Autodesk Inventor part; units mm, degrees
ref_plane "Płaszczyzna konstrukcyjna1" through (0, 15, 0) normal (0, 1, 0) x (-1, 0, 0)
ref_plane "YZ Plane" through (0, 0, 0) normal (1, 0, 0) x (0, 1, 0)
ref_plane "XY Plane" through (0, 0, 0) normal (0, 0, 1) x (1, 0, 0)
sketch "Szkic1" plane through (0, 0, 0) normal (0, 1, 0) x (-1, 0, 0)
  line L0 (15, 0) -> (-15, 0)
  line L1 (-15, 0) -> (-15, -600)
  line L2 (-15, -600) -> (15, -600)
  line L3 (15, -600) -> (15, 0)
  point P0 (0, 0)
  point P1 (0, 0)
  dimension "d0" = 30
  dimension "d1" = 600
extrude "Wyciągnięcie proste1" add sketch "Szkic1" along normal blind 30
sketch "Szkic2" plane through (-15, 0, 0) normal (0, 0, 1) x (1, 0, 0)
  line L0 (0, 0) -> (0, 30)
  line L1 (0, 0) -> (30, 0)
  line L2 (30, 0) -> (30, 30)
  line L3 (0, 30) -> (30, 30)
  line L4 (0, 0) -> (0, 30)
  line L5 (0, -15) -> (30, -15)
  line L6 (30, -15) -> (30, 45)
  line L7 (30, 45) -> (0, 45)
  line L8 (0, 45) -> (0, -15)
  point P0 (15, 0)
  point P1 (0, 15)
  point P2 (0, 15)
  dimension "d4" = 60
  dimension "d5" = 30
extrude "Wyciągnięcie proste2" add sketch "Szkic2" along normal blind 10
sketch "Szkic3" plane through (-15, 0, 10) normal (0, 0, 1) x (1, 0, 0)
  line L0 (0, -15) -> (30, -15)
  line L1 (30, -15) -> (30, 45)
  line L2 (0, -15) -> (30, -15)
  line L3 (30, -15) -> (30, 0)
  line L4 (30, 0) -> (0, 0)
  line L5 (0, 0) -> (0, -15)
  point P0 (15, 0)
extrude "Wyciągnięcie proste3" add sketch "Szkic3" along normal blind 60
ref_plane "Płaszczyzna konstrukcyjna1" through (0, 15, 0) normal (0, 1, 0) x (-1, 0, 0)
mirror "Odbicie lustrzane1" about plane through (0, 15, 0) normal (0, 1, 0) of "Wyciągnięcie proste3"
sketch "Szkic4" plane through (0, 15, 0) normal (0, 1, 0) x (-1, 0, 0)
  point P0 (0, 0)
sketch "Szkic5" plane through (-15, 45, 0) normal (0, 1, 0) x (1, 0, 0)
  line L0 (0, -70) -> (30, -70)
  line L1 (30, 0) -> (30, -70)
  circle A0 centre (15, -50) radius 7.5
  point P0 (15, 0)
  dimension "d11" = 15
  dimension "d12" = 20
  dimension "d13" = 15
extrude "Wyciągnięcie proste4" cut sketch "Szkic5" against normal through all
fillet "Zaokrąglenie1" radius 4 12 edges at (0, 45, 0) (0, 45, 70) (0, 0, 70) (-15, 0, -300) (-15, 30, -300) (-15, 15, -600) (0, 0, -600) (0, 30, -600) (15, 15, -600) (15, 0, -300) (15, 30, -300) (0, -15, 0)
sketch "Szkic6" plane through (0, 0, 0) normal (0, -1, 0) x (1, 0, 0)
  circle A0 centre (0, -580) radius 10
  line L0 (-11, -600) -> (11, -600)
  line L1 (-15, 0) -> (-15, -596)
  point P0 (0, 0)
  dimension "d17" = 20
  dimension "d18" = 20
  dimension "d19" = 15
extrude "Wyciągnięcie proste5" cut sketch "Szkic6" against normal through all
fillet "Zaokrąglenie2" radius 4 3 edges at (0, -15, 70) (15, -3.5, 0) (-15, -3.5, 0)
fillet "Zaokrąglenie3" radius 4 1 edges at (0, 30, 70)
properties part number "2" material "Złote"
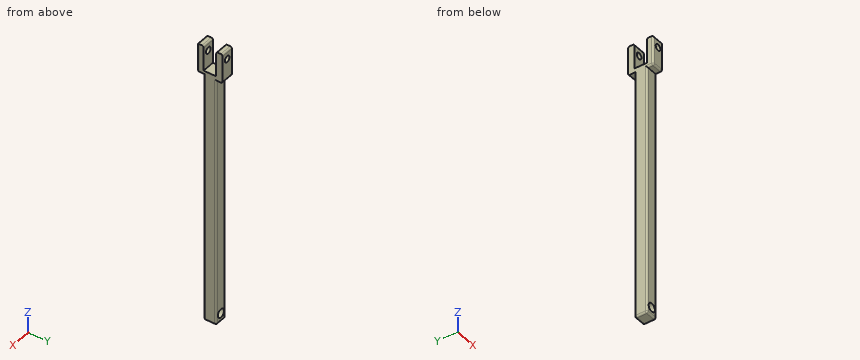
Can you work these out from the model? Positions are in its coordinate system, mm. Give positions to 0.01 mm unless a question says otherwise; leave off trailing zeros. Loops run counter-clockwise (first coordinate to the right, second up) from the corner with the lowest first, then second, coordinate; pieces in that order, holes last. Notation, with made-up numbers: (-36.5, -6) -> (5.5, -6) arc R22 ccw to (5.5, 23) -> close; hole circle Ø3 at (86, 37). An arc over 180 degrees is marked (long way). Use one line per item in the form item = value.
1) Will these pins go through, and if not, where does the flat tip stop? pin 1 (10 mm diameter, centred on x = 2.5, y = -3.5, fed in from -Z); pin 2 (9 mm diameter, centred on x = -5.5, y = 9, fed in from +Z); pin 3 (4 mm diameter, centred on x = 5, z = -88, fed in from -Y).
Answers:
pin_1 = -599.12
pin_2 = 10
pin_3 = 0
2) If we section it at A-A (z = 50): Please give me the cut outline in (x, y).
Answers:
outline = (-15, -11) arc R4 ccw to (-11, -15) -> (-7.5, -15) -> (-7.5, 0) -> (-15, 0) -> close; (-15, 30) -> (-7.5, 30) -> (-7.5, 45) -> (-15, 45) -> close; (7.5, -15) -> (11, -15) arc R4 ccw to (15, -11) -> (15, 0) -> (7.5, 0) -> close; (7.5, 30) -> (15, 30) -> (15, 45) -> (7.5, 45) -> close
3) If we section it at C-C (y = 18): Please give me the cut outline in (x, z).
Answers:
outline = (-15, -596) arc R4 ccw to (-11, -600) -> (11, -600) arc R4 ccw to (15, -596) -> (15, 10) -> (-15, 10) -> close; hole circle Ø20 at (0, -580)
4) If we section it at D-D (z = -580): Please give me the cut outline in (x, y).
Answers:
outline = (-15, 4) arc R4 ccw to (-11, 0) -> (-10, 0) -> (-10, 30) -> (-11, 30) arc R4 ccw to (-15, 26) -> close; (10, 0) -> (11, 0) arc R4 ccw to (15, 4) -> (15, 26) arc R4 ccw to (11, 30) -> (10, 30) -> close
5) I need wall thicknesses on line 1 along Z through (x, y) = (0, 39.75); line 2 along Z through (x, y) = (0, 8); line 3 along Y through (x, z) = (-10.25, 38). Which ranges of each line are inside material? Lowest first, please.
Answers:
line_1 = 0 to 42.5, 57.5 to 70
line_2 = -600 to -590, -570 to 10
line_3 = -15 to 0, 30 to 45
6) If we section it at B-B (x = 0): Count the separate pieces of the cut face and the enclosed holes in it, plus the area to 3 significant figures.
Answers:
separate_pieces = 4
enclosed_holes = 0
area = 19,300 mm²
